Source: CAD feature listing. Evaluate the final solid. Frame: model axes, mm. Face numbers are marked on the shaded views. A direction names the side the tool comes from. Round coordinates to 2 decimals unless told otherwise and drop trailing zeros. Order: outer loops, then holes, each group sorted by start corner. A loop starts at its lowest first (then second) coordinate and runs counter-clockwise, first axis right, second up. Notation, with made-up numbers: M 8.25,65 L 21.25,65 A7 cw 21.25,75 Z; hole C 87.5,44.5 d2. An arc over 180 degrees is marked long. Answer as CSV lines item,"result". Start each with the question number.
Item 1: Section query C-C on x = 23. Return the cut outline in (y, z), plus the area to 3 significant figures.
Item 2: Set-up query: the marked faces 1 and 2. Return all of +Z, -Z, +X, -X, +Y, -Y with unobstructed straight access to the full face (end or side cutting, diameter ignored); none if empty.
Item 3: Section query D-D on z = 112. Return the cut outline in (x, y).
Item 4: First-contact query: P1, Ø6, axis at y = 4, z = 107.5, coming from the +X side; P2, Ø12, axis at y = 16, z = 75.5, coming from the +X side; P3, Ø9, axis at y = -8, z = 0, coming from the -X side. Flat tips, straight axial feed; report the tip coordinate or a pass-through.
Item 5: Line query: line 1 (X direction, y = 18, z = -1); line 2 (Y direction, x = 35, z = 0). Output: solid intervals per line, ascending. Write a range as [from, to].
Item 6: Section query A-A on y = -7.25. Return the cut outline in (x, z), plus the area to 3 significant figures.
Item 7: Section query B-B on y = -28. Return the cut outline in (x, z), plus the area to 3 significant figures.
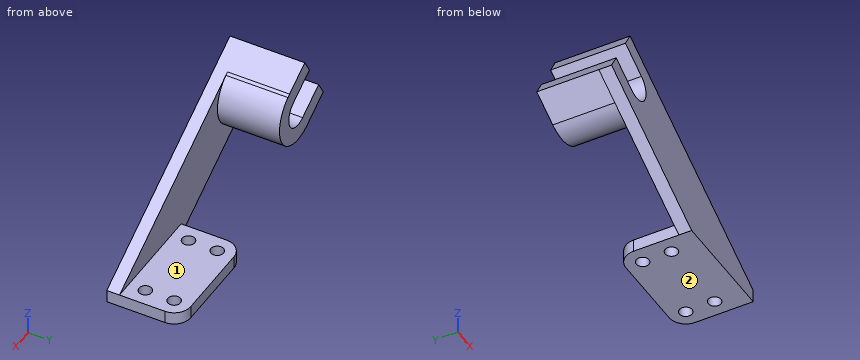
from build123d import *

# Parameters (mm, degrees)
SKETCH_1_W                = 100
SKETCH_1_H                = 67.5
EXTRUDE_1_DEPTH           = 5.75
FILLET_1_R                = 15
HOLE_WIZARD_11_5_11_5_1_D = 11.5
EXTRUDE_2_DEPTH           = 11.5
EXTRUDE_3_DEPTH           = 56


with BuildPart() as part:
    # 草图1 → 凸台-拉伸1 (new, symmetric)
    with BuildSketch(Plane.XY):
        Rectangle(SKETCH_1_W, SKETCH_1_H)
    extrude(amount=EXTRUDE_1_DEPTH, both=True)

    # 圆角1
    fillet_1_edges = [part.edges().sort_by_distance(p)[0] for p in [
        (-50, 33.75, 0),
        (50, 33.75, 0),
    ]]
    fillet(fillet_1_edges, radius=FILLET_1_R)

    # Ø11.5 (11.5) 直径孔1 (through all)
    with Locations(Plane.XY.offset(5.75)):
        with Locations((-35, 18.75), (35, 18.75), (-35, -7.25), (35, -7.25)):
            Hole(HOLE_WIZARD_11_5_11_5_1_D / 2)

    # 草图5 → 凸台-拉伸2 (add)
    with BuildSketch(Plane.XZ.offset(33.75)):
        with BuildLine():
            Line((-179.903810568, 69.25), (-50, -5.75))
            Line((-50, -5.75), (-50, 5.75))
            Line((-50, 5.75), (50, 5.75))
            Line((50, 5.75), (-149.924164496, 121.176270189))
            Line((-149.924164496, 121.176270189), (-157.403810568, 108.22114317))
            Line((-157.403810568, 108.22114317), (-131.423048454, 93.22114317))
            ThreePointArc((-131.423048454, 93.22114317), (-125.932667397, 72.730762114), (-146.423048454, 67.240381057))
            Line((-146.423048454, 67.240381057), (-172.403810568, 82.240381057))
            Line((-172.403810568, 82.240381057), (-179.903810568, 69.25))
        make_face()
    extrude(amount=-EXTRUDE_2_DEPTH)

    # 草图6 → 凸台-拉伸3 (add)
    with BuildSketch(Plane(origin=(0, -22.25, 0), x_dir=(1, 0, 0), z_dir=(0, 1, 0))):
        with BuildLine():
            Line((-125.296403009, -106.957425465), (-122.590401756, -105.395114913))
            ThreePointArc((-122.590401756, -105.395114913), (-113.341811547, -64.559121538), (-153.923048454, -54.25))
            Line((-153.923048454, -54.25), (-179.903810568, -69.25))
            Line((-179.903810568, -69.25), (-172.403810568, -82.240381057))
            Line((-172.403810568, -82.240381057), (-146.423048454, -67.240381057))
            ThreePointArc((-146.423048454, -67.240381057), (-125.932667397, -72.730762114), (-131.423048454, -93.22114317))
            Line((-131.423048454, -93.22114317), (-157.403810568, -108.22114317))
            Line((-157.403810568, -108.22114317), (-149.924164496, -121.176270189))
            Line((-149.924164496, -121.176270189), (-125.296403009, -106.957425465))
        make_face()
    extrude(amount=EXTRUDE_3_DEPTH)


solid = part.part
Results:
1,outline,"M -33.75,-5.75 L 33.75,-5.75 L 33.75,5.75 L -22.25,5.75 L -22.25,21.34 L -33.75,21.34 Z"
1,area,"956 mm^2"
2,face 1,"+Z, +X, -X, +Y"
2,face 2,"-Z, +X, -X, +Y, -Y"
3,outline,"M -155.22,-33.75 L -134.03,-33.75 L -134.03,33.75 L -155.22,33.75 Z"
4,P1,"x = -121.29"
4,P2,"x = -108.92"
4,P3,"x = -50"
5,line 1,"[-50, -40.7], [-29.3, 29.3], [40.7, 50]"
5,line 2,"[-33.75, -13], [-1.5, 13], [24.5, 33.75]"
6,outline,"M -179.9,69.25 L -153.92,54.25 A30 ccw -122.59,105.4 L -149.92,121.18 L -157.4,108.22 L -131.42,93.22 A15 cw -146.42,67.24 L -172.4,82.24 Z; M -50,-5.75 L -40.75,-5.75 L -40.75,5.75 L -50,5.75 Z; M -29.25,-5.75 L 29.25,-5.75 L 29.25,5.75 L -29.25,5.75 Z; M 40.75,-5.75 L 50,-5.75 L 50,5.75 L 40.75,5.75 Z"
6,area,"2,840 mm^2"
7,outline,"M -179.9,69.25 L -50,-5.75 L 50,-5.75 L 50,5.75 L -149.92,121.18 L -157.4,108.22 L -131.42,93.22 A15 cw -146.42,67.24 L -172.4,82.24 Z"
7,area,"10,700 mm^2"
